For this review, use the dimensioned drawing (mm, ordinates from the lowest corner) and the shaded views. Coordinates: 2 decimals unless noted, no trailing zeros. Loops run counter-clockwise (first coordinate to the right, second up) from the corner with the lowest first, then second, coordinate; pieces in that order, holes last. Notation, with made-up numbers: (-11.75, -33.75) - (36.25, -33.75) arc R12 ccw to (36.25, -11.75) - close; hole circle Ø7 at (79.5, 49). An arc over 180 degrees is marked (long way). Use a Markdown table: item, result. Add a question column.
1) Add section B-B, the plane x = 67.82. Give the boundary of the cut face in (y, z).
2) To check wall thickness, follow L1, parallel to Y at x = 67.82, z = 7.95; L2, parallel to Y at x = 67.82, z = 2. State the ranges of each line that lie inside material, in increasing order. Write a range as [from, to].
3) Add section A-A, the plane y = 28.32. Give the boundary of the cut face in (x, z), and give its area (3 significant figures).
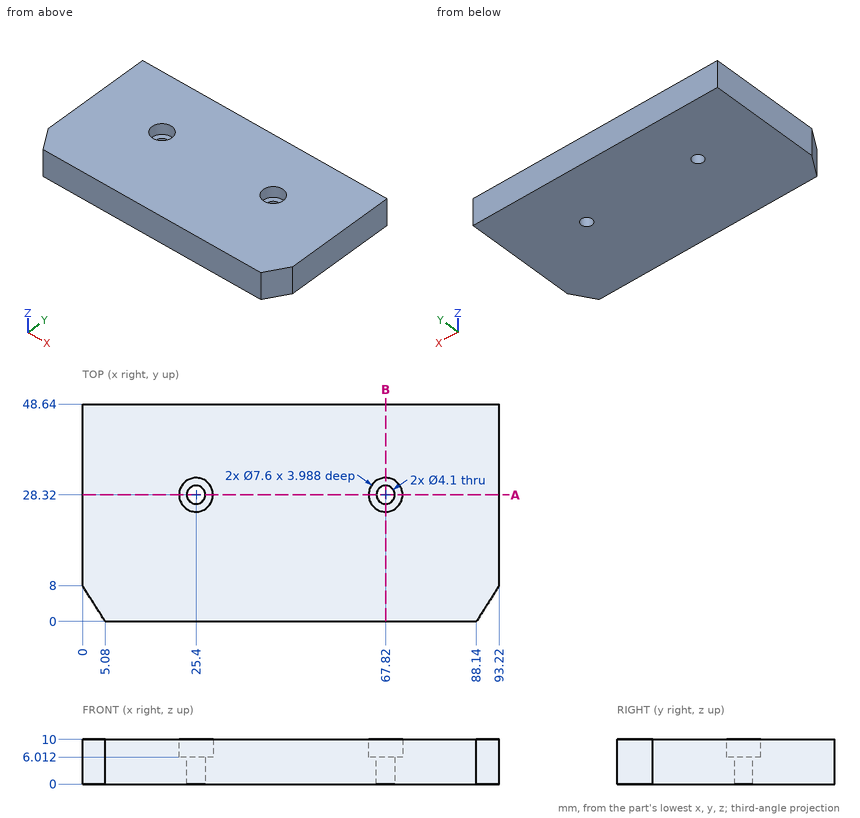
From the geometry:
| question | item | result |
|---|---|---|
| 1 | outline | (0, 0) - (26.27, 0) - (26.27, 6.01) - (24.52, 6.01) - (24.52, 10) - (0, 10) - close; (30.37, 0) - (48.64, 0) - (48.64, 10) - (32.12, 10) - (32.12, 6.01) - (30.37, 6.01) - close |
| 2 | L1 | y = [0, 24.52], [32.12, 48.64] |
| 2 | L2 | y = [0, 26.27], [30.37, 48.64] |
| 3 | outline | (0, 0) - (23.35, 0) - (23.35, 6.01) - (21.6, 6.01) - (21.6, 10) - (0, 10) - close; (27.45, 0) - (65.77, 0) - (65.77, 6.01) - (64.02, 6.01) - (64.02, 10) - (29.2, 10) - (29.2, 6.01) - (27.45, 6.01) - close; (69.87, 0) - (93.22, 0) - (93.22, 10) - (71.62, 10) - (71.62, 6.01) - (69.87, 6.01) - close |
| 3 | area | 822 mm^2 |
